Geometry: final body of the model. Coordinates: model frame, mm. Face numbers are marked on the shaded views. Round coordinates to 2 decimals unless told otherwise and drop trailing zeros. Loops run counter-clockwise (first coordinate to the right, second up) from the corner with the lowest first, then second, coordinate; pieces in that order, holes last. Notation, with made-up numbers: M 75.5,31 L 88.5,31 A7 cw 88.5,38 Z; hole C 35.25,83.25 d1. An arc over 180 degrees is marked long. Answer as a JSON object with one key per item and string values.
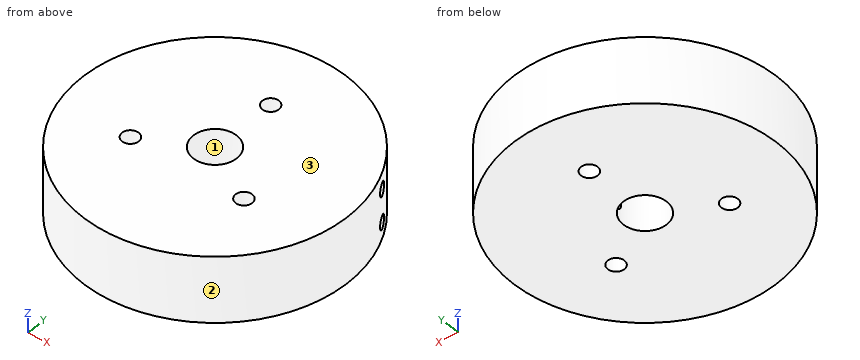
```python
from build123d import *

# Parameters (mm, degrees)
SKETCH1_R                           = 20
SKETCH1_R_2                         = 1.250479472
SKETCH1_R_3                         = 3.275
BOSS_EXTRUDE1_DEPTH                 = 10
CUT_EXTRUDE2_REACH                  = 41.275
CUT_EXTRUDE2_END_RADIUS             = 20
SKETCH4_R                           = 1
CUT_EXTRUDE2_DIRECTION_2_REACH      = 41.275
CUT_EXTRUDE2_DIRECTION_2_END_RADIUS = 3.275


with BuildPart() as part:
    # Sketch1 → Boss-Extrude1 (new body)
    with BuildSketch(Plane.XY):
        Circle(SKETCH1_R)
        with Locations((0, 10)):
            Circle(SKETCH1_R_2, mode=Mode.SUBTRACT)
        Circle(SKETCH1_R_3, mode=Mode.SUBTRACT)
        with Locations((8.660254038, -5)):
            Circle(SKETCH1_R_2, mode=Mode.SUBTRACT)
        with Locations((-8.660254038, -5)):
            Circle(SKETCH1_R_2, mode=Mode.SUBTRACT)
    extrude(amount=BOSS_EXTRUDE1_DEPTH)

    # Cut-Extrude2: up to this cylinder (the profile starts inside it)
    cut_extrude2_end = Plane(origin=(0, 0, 5), z_dir=(0, 0, -1)) * Cylinder(CUT_EXTRUDE2_END_RADIUS, 128.55, mode=Mode.PRIVATE)
    # Sketch4 → Cut-Extrude2 (cut, up to the surface)
    with BuildSketch(Plane(origin=(8.979891602, 4.550503837, 0), x_dir=(0.4520194972044375, -0.8920080572209242, 0), z_dir=(-0.8920080572209242, -0.4520194972044375, 0)), mode=Mode.PRIVATE) as cut_extrude2_sk1:
        with Locations(Location((0, 7.5, 0), (0, 0, 180))):
            Circle(SKETCH4_R)
    cut_extrude2_tool1 = extrude(cut_extrude2_sk1.sketch, amount=-CUT_EXTRUDE2_REACH, mode=Mode.PRIVATE) & cut_extrude2_end
    add(cut_extrude2_tool1.solids().sort_by_distance((8.979892, 4.550504, 7.5))[0], mode=Mode.SUBTRACT)
    # Sketch4 → Cut-Extrude2 (cut, up to the surface)
    with BuildSketch(Plane(origin=(8.979891602, 4.550503837, 0), x_dir=(0.4520194972044375, -0.8920080572209242, 0), z_dir=(-0.8920080572209242, -0.4520194972044375, 0)), mode=Mode.PRIVATE) as cut_extrude2_sk2:
        with Locations(Location((0, 2.5, 0), (0, 0, 180))):
            Circle(SKETCH4_R)
    cut_extrude2_tool2 = extrude(cut_extrude2_sk2.sketch, amount=-CUT_EXTRUDE2_REACH, mode=Mode.PRIVATE) & cut_extrude2_end
    add(cut_extrude2_tool2.solids().sort_by_distance((8.979892, 4.550504, 2.5))[0], mode=Mode.SUBTRACT)

    # Cut-Extrude2 direction 2: up to this cylinder (the profile starts outside it)
    cut_extrude2_direction_2_end = Plane(origin=(0, 0, 5), z_dir=(0, 0, -1)) * Cylinder(CUT_EXTRUDE2_DIRECTION_2_END_RADIUS, 95.1, mode=Mode.PRIVATE)
    # Sketch4 → Cut-Extrude2 direction 2 (cut, up to the surface)
    with BuildSketch(Plane(origin=(8.979891602, 4.550503837, 0), x_dir=(0.4520194972044375, -0.8920080572209242, 0), z_dir=(-0.8920080572209242, -0.4520194972044375, 0)), mode=Mode.PRIVATE) as cut_extrude2_direction_2_sk1:
        with Locations(Location((0, 7.5, 0), (0, 0, 180))):
            Circle(SKETCH4_R)
    cut_extrude2_direction_2_tool1 = extrude(cut_extrude2_direction_2_sk1.sketch, amount=CUT_EXTRUDE2_DIRECTION_2_REACH, mode=Mode.PRIVATE) - cut_extrude2_direction_2_end
    add(cut_extrude2_direction_2_tool1.solids().sort_by_distance((8.979892, 4.550504, 7.5))[0], mode=Mode.SUBTRACT)
    # Sketch4 → Cut-Extrude2 direction 2 (cut, up to the surface)
    with BuildSketch(Plane(origin=(8.979891602, 4.550503837, 0), x_dir=(0.4520194972044375, -0.8920080572209242, 0), z_dir=(-0.8920080572209242, -0.4520194972044375, 0)), mode=Mode.PRIVATE) as cut_extrude2_direction_2_sk2:
        with Locations(Location((0, 2.5, 0), (0, 0, 180))):
            Circle(SKETCH4_R)
    cut_extrude2_direction_2_tool2 = extrude(cut_extrude2_direction_2_sk2.sketch, amount=CUT_EXTRUDE2_DIRECTION_2_REACH, mode=Mode.PRIVATE) - cut_extrude2_direction_2_end
    add(cut_extrude2_direction_2_tool2.solids().sort_by_distance((8.979892, 4.550504, 2.5))[0], mode=Mode.SUBTRACT)


solid = part.part
```
1) Line query: probe 1 along Y at (x, z) = (0, 2.75) (3 decimals); probe 2 along X at (y, z) = (-4, 4); probe 3 along X at (y, z) = (3, 7.5). Output: solid intervals per line, ascending.
Geometry results:
{"probe 1": "-20 to -3.275, 3.275 to 8.75, 11.25 to 20", "probe 2": "-19.6 to -9.41, -7.91 to 7.91, 9.41 to 19.6", "probe 3": "-19.77 to -1.31, 1.31 to 3.71, 8.13 to 19.77"}
2) First-contact query: pin 1 (1 mm diameter, centred on x = 6.5, z = 8, fed in from -Y); pin 2 (5 mm diameter, centred on y = -3, z = 5.5, fed in from -X); pin 3 (1 mm diameter, centred on x = 4.5, z = 6, fed in from -Y). Flat tips, straight axial feed; report the tip coordinate or a pass-through.
Geometry results:
{"pin 1": "y = -19.08", "pin 2": "x = -19.99", "pin 3": "y = -19.6"}
3) Pull-direction query (X, two-part tool) for the marked faces 1, 2 and 3; classes: +X half, -X half, draft (parallel to the pull), parting line (faces both ways), or undercut.
Geometry results:
{"face 1": "undercut", "face 2": "parting line", "face 3": "draft"}
4) Cut plane A-A on x = 0. Return the cut outline in (y, z) (3 decimals).
Geometry results:
{"outline": "M -20,0 L -3.275,0 L -3.275,10 L -20,10 Z; M 3.275,0 L 8.75,0 L 8.75,10 L 3.275,10 Z; M 11.25,0 L 20,0 L 20,10 L 11.25,10 Z"}
5) Cut plane B-B on y = 0. Return the cut outline in (x, z) (3 decimals), and give its area (4 significant figures).
Geometry results:
{"outline": "M -20,0 L -3.275,0 L -3.275,10 L -20,10 Z; M 3.275,0 L 20,0 L 20,10 L 3.275,10 Z", "area": "334.5 mm2"}
6) Cut plane D-D on y = -5. Return the cut outline in (x, z).
Geometry results:
{"outline": "M -19.36,0 L -9.91,0 L -9.91,10 L -19.36,10 Z; M -7.41,0 L 7.41,0 L 7.41,10 L -7.41,10 Z; M 9.91,0 L 19.36,0 L 19.36,10 L 9.91,10 Z"}
7) Cut plane C-C on z = 5.5. Return the cut outline in (x, y) (3 decimals), and give its area (3 significant figures).
Geometry results:
{"outline": "C 0,0 d40; hole C -8.66,-5 d2.501; hole C 0,0 d6.55; hole C 0,10 d2.501; hole C 8.66,-5 d2.501", "area": "1,210 mm2"}
